Here's how the part is built. I have some questions about the finished solid (model axes, mm). A direction names the side the tool comes from. Coordinates: 2 decimals unless noted, no trailing zeros. Write each loop counter-clockwise with the first axis right and the second up, starting at its lowest first coordinate (ties: lowest second). Pieces come first, ordered by that corner, then holes.
Item 1: If I drill on line 1 (Y direction, x = 2.5, z = 1.5); line 2 (X direction, y = 20, z = 12.25); line 3 (Z direction, x = 3, y = 26.5), over which ranges is the centre line in solid material (lowest first)?
Item 2: I'm going to push flat-ended pins straight in: pin 1 Ø6 at (x, y) = (19, 24.5) entering from -Z; pin 2 Ø1.2 at (x, y) = (13, 40) entering from -Z. Where does each tip first touch, or does it pass through?
Item 3: For faces 5 (the face through (5.679, 40, 5)), 6 (the face through (20.01, 17.6, 11.73)), 7 (the face through (1, 20, 9.832)), which set-ups out of +Z, -Z, +X, -X, +Y, -Y let a thin tool reach every point of the face, with its end or its side?
Item 4: If we section it at B-B (x = 7): Please give me the cut outline in (y, z).
Item 5: We'd pull the mould along Y, two halves only. Please class faces 1 (the face through (25.647, 40, 5)), 2 (the face through (16, 41, 11)), 3 (the face through (16.984, 20.382, 11.732)), 4 (the face through (1, 37.702, 5)): +Y half, -Y half, draft (parallel to the pull), parting line (faces both ways), or undercut.
Item 6: If we section it at C-C (y = 16): Please give me the cut outline in (x, z), then the cut area to 3 significant figures.
Item 7: If we section it at A-A (z = 7.25): Please give me the cut outline in (x, y).
Item 8: If we section it at D-D (x = 14.5): Please give me the cut outline in (y, z).
Autodesk Fusion 360 part; units mm, degrees
sketch "Sketch1" plane through (0, 0, 0) normal (0, 0, 1) x (1, 0, 0)
  line L0 (0, 0) -> (31, 0)
  line L1 (31, 0) -> (31, 41)
  line L2 (31, 41) -> (0, 41)
  line L3 (0, 41) -> (0, 0)
  line L4 (1.5, 39.5) -> (29.5, 39.5)
  line L5 (29.5, 39.5) -> (29.5, 1.5)
  line L6 (29.5, 1.5) -> (1.5, 1.5)
  line L7 (1.5, 1.5) -> (1.5, 39.5)
  line L8 (1.5, 39.5) -> (29.5, 1.5) construction
  line L9 (29.5, 39.5) -> (1.5, 1.5) construction
  circle A0 centre (15.5, 28.7333) radius 7.5
  point P0 (15.5, 20.5)
  dimension "d1" = 31
  dimension "d2" = 41
  dimension "d3" = 28
  dimension "d4" = 38
  dimension "d5" = 15
extrude "Extrude1" add sketch "Sketch1" along normal blind 2 contours L0 L1 L2 L3 | L4 L5 L6 L7 makes body 1
extrude "Extrude2" add sketch "Sketch1" along normal blind 4 contours L4 L5 L6 L7 bodies 1
sketch "Sketch1 (2)" plane through (0, 0, 2) normal (0, 0, 1) x (-1, 0, 0) in component "Top"
  line L0 (-1.5, -1.5) -> (-1.5, -39.5)
  line L1 (-1.5, -39.5) -> (-29.5, -39.5)
  line L2 (-29.5, -39.5) -> (-29.5, -1.5)
  line L3 (-29.5, -1.5) -> (-1.5, -1.5)
  line L4 (0, -41) -> (0, 0)
  line L5 (0, 0) -> (-31, 0)
  line L6 (-31, 0) -> (-31, -41)
  line L7 (-31, -41) -> (0, -41)
  line L8 (0, -41) -> (-31, -41)
  line L9 (-31, -41) -> (-31, 0)
  line L10 (-31, 0) -> (0, 0)
  line L11 (0, 0) -> (0, -41)
extrude "Extrude1'" add sketch "Sketch1 (2)" along normal blind 10 separate body contours L0 L1 L2 L3 | L4 L5 L6 L7 L8 L9 L10 L11 makes body 2 in component "Top"
shell "Shell1" thickness 1.5 removed faces 1 at (10.3333, 27.3333, 2) on bodies 2 in component "Top"
ref_plane "WorkPlane1" through (15.5, 20.5, 12) normal (0, 0, 1) x (1, 0, 0)
sketch "Sketch2" plane through (15.5, 20.5, 12) normal (0, 0, 1) x (1, 0, 0) in component "Top"
  line L0 (0.1136, 9.8824) -> (-8.6176, 4.8413)
  line L1 (-8.6176, 4.8413) -> (-8.6176, -5.2393)
  line L2 (-8.6176, -5.2393) -> (0.1136, -10.2796)
  line L3 (0.1136, -10.2796) -> (8.8449, -5.2393)
  line L4 (8.8449, -5.2393) -> (8.8449, 4.8413)
  line L5 (8.8449, 4.8413) -> (0.1136, 9.8824)
  line L6 (-2.4502, 5.2787) -> (0.1835, 5.2787)
  line L7 (0.1835, 5.2787) -> (-3.4193, -0.2014)
  line L8 (-3.4193, -0.2014) -> (-6.053, -0.2014)
  line L9 (-6.053, -0.2014) -> (-2.4502, 5.2787)
  line L10 (-4.8021, -5.6751) -> (2.4028, 5.2866)
  line L11 (2.4028, 5.2866) -> (5.0365, 5.2866)
  line L12 (5.0365, 5.2866) -> (-2.1692, -5.6751)
  line L13 (-2.1692, -5.6751) -> (-4.8021, -5.6751)
  line L14 (2.6854, -5.6751) -> (0.0517, -5.6751)
  line L15 (0.0517, -5.6751) -> (3.6538, -0.195)
  line L16 (3.6538, -0.195) -> (6.2874, -0.195)
  line L17 (6.2874, -0.195) -> (2.6854, -5.6751)
extrude "Extrude2'" cut sketch "Sketch2" against normal blind 0.5 bodies 2 in component "Top"
extrude "Extrude3" cut 3 faces at (19.7089, 18.4783, 12) (17.2567, 22.1327, 12) (13.6047, 23.952, 12) along direction (0, 0, -1) blind 2 on bodies 2 bodies 2 in component "Top"
sketch "Sketch2 (1)" plane through (0, 41, 0) normal (0, 1, 0) x (-1, 0, 0) in component "Top"
  line L0 (-31, 2) -> (0, 2)
  line L1 (0, 2) -> (0, 12)
  line L2 (0, 12) -> (-31, 12)
  line L3 (-31, 12) -> (-31, 2)
  line L4 (-28.0584, 2) -> (-2.1668, 2)
  line L5 (-2.1668, 2) -> (-2.1668, 9.9165)
  line L6 (-2.1668, 9.9165) -> (-28.0584, 9.9165)
  line L7 (-28.0584, 9.9165) -> (-28.0584, 2)
  point P0 (-15.5, 7)
sketch "Sketch3" plane through (31, 0, 0) normal (1, 0, 0) x (0, 1, 0) in component "Top"
  line L0 (0, 2) -> (41, 2)
  line L1 (41, 2) -> (41, 12)
  line L2 (41, 12) -> (0, 12)
  line L3 (0, 12) -> (0, 2)
  line L4 (3.2975, 9.8315) -> (37.7025, 9.8315)
  line L5 (37.7025, 9.8315) -> (37.7025, 4.1685)
  line L6 (37.7025, 4.1685) -> (3.2975, 4.1685)
  line L7 (3.2975, 4.1685) -> (3.2975, 9.8315)
  line L8 (3.2975, 9.8315) -> (37.7025, 4.1685) construction
  line L9 (37.7025, 9.8315) -> (3.2975, 4.1685) construction
  point P0 (20.5, 7)
extrude "Extrude5" cut sketch "Sketch3" against normal blind 35 contours L4 L5 L6 L7 bodies 2 in component "Top"
extrude "Extrude6" add 1 faces at (15.5379, 37.4608, 12) along direction (0, 0, 1) blind 1 on bodies 2 bodies 2 in component "Top"
extrude "Extrude7" add 1 faces at (9.7931, 23.8062, 11.5) along direction (0, 0, 1) blind 1.5 on bodies 2 bodies 2 in component "Top"
extrude "Extrude8" cut 1 faces at (15.5612, 35.9262, 13) along direction (0, 0, 1) blind 1 on bodies 2 bodies 2 in component "Top"
extrude "Extrude9" add sketch "Sketch1 (2)" against normal blind 2.5 bodies 2 in component "Top"
sketch "Sketch4" plane through (0, 0, 0) normal (-1, 0, 0) x (0, -1, 0) in component "Top"
  line L0 (-37.7025, 4.1685) -> (-37.7025, 9.8315)
  line L1 (-37.7025, 9.8315) -> (-3.2975, 9.8315)
  line L2 (-3.2975, 9.8315) -> (-3.2975, 4.1685)
  line L3 (-3.2975, 4.1685) -> (-37.7025, 4.1685)
  line L4 (0, -0.5) -> (0, 13)
  line L5 (0, 13) -> (-41, 13)
  line L6 (-41, 13) -> (-41, -0.5)
  line L7 (-41, -0.5) -> (0, -0.5)
  line L8 (-37.7025, 9.8315) -> (-3.2975, 9.8315)
  line L9 (-3.2975, 9.8315) -> (-3.2975, -1.832)
  line L10 (-3.2975, -1.832) -> (-37.7025, -1.832)
  line L11 (-37.7025, -1.832) -> (-37.7025, 9.8315)
extrude "Extrude10" cut sketch "Sketch4" against normal blind 45.044 contours L0 L1 L2 L3 L8 L9 L11 | L3 L7 L9 L11 | L7 L9 L10 L11 bodies 2 in component "Top"
sketch "Sketch5" plane through (0, 0, 0) normal (0, -1, 0) x (1, 0, 0) in component "Top"
  line L0 (31, -0.5) -> (31, 13)
  line L1 (31, 13) -> (0, 13)
  line L2 (0, 13) -> (0, -0.5)
  line L3 (0, -0.5) -> (31, -0.5)
  line L4 (5.6791, -0.5) -> (25.6474, -0.5)
  line L5 (25.6474, -0.5) -> (25.6474, 9.8926)
  line L6 (25.6474, 9.8926) -> (5.6791, 9.8926)
  line L7 (5.6791, 9.8926) -> (5.6791, -0.5)
extrude "Extrude11" cut sketch "Sketch5" against normal blind 159.301 contours L3 L4 L5 L6 L7 bodies 2 in component "Top"
component "Top" placed x (1, 0, 0) y (0, 1, 0) z (0, 0, 1) at (0, 0, 0)
hidden bodies 1
Answer list:
1. line 1: y = 0 to 1.5, 39.5 to 41
1. line 2: x = 0 to 14.1, 16.73 to 18.95, 21.59 to 31
1. line 3: z = 10.5 to 13
2. pin 1: stops at z = 10.5
2. pin 2: stops at z = 9.89
3. face 5: -Z, +Y, -Y
3. face 6: +Z, -Z
3. face 7: -Z, +X, -X
4. outline: (0, 9.89) - (1.5, 9.89) - (1.5, 10.5) - (39.5, 10.5) - (39.5, 9.89) - (41, 9.89) - (41, 13) - (0, 13) - close
5. face 1: draft
5. face 2: +Y half
5. face 3: undercut
5. face 4: undercut
6. outline: (0, 9.83) - (1.5, 9.83) - (1.5, 10.5) - (11.47, 10.5) - (11.47, 13) - (0, 13) - close; (14.1, 10.5) - (16.32, 10.5) - (16.32, 13) - (14.1, 13) - close; (18.96, 10.5) - (29.5, 10.5) - (29.5, 9.83) - (31, 9.83) - (31, 13) - (18.96, 13) - close
6. area: 66.3 mm2
7. outline: (0, 0) - (5.68, 0) - (5.68, 1.5) - (1.5, 1.5) - (1.5, 3.3) - (0, 3.3) - close; (0, 37.7) - (1.5, 37.7) - (1.5, 39.5) - (5.68, 39.5) - (5.68, 41) - (0, 41) - close; (25.65, 0) - (31, 0) - (31, 3.3) - (29.5, 3.3) - (29.5, 1.5) - (25.65, 1.5) - close; (25.65, 39.5) - (29.5, 39.5) - (29.5, 37.7) - (31, 37.7) - (31, 41) - (25.65, 41) - close
8. outline: (0, 9.89) - (1.5, 9.89) - (1.5, 10.5) - (16.6, 10.5) - (16.6, 13) - (0, 13) - close; (20.61, 10.5) - (23.98, 10.5) - (23.98, 13) - (20.61, 13) - close; (25.78, 10.5) - (39.5, 10.5) - (39.5, 9.89) - (41, 9.89) - (41, 13) - (25.78, 13) - close
